```python
from build123d import *

# Parameters (mm, degrees)
F1_DEPTH = 26
F3_DEPTH = 2


with BuildPart() as f1:
    # F0 (on Top) → F1 (new body, symmetric)
    with BuildSketch(Plane.XY):
        with BuildLine():
            Line((-21.6270365771, 1), (-21.6270365771, 0))
            Line((-21.6270365771, 0), (-13.1270365771, 0))
            ThreePointArc((-13.1270365771, 0), (1.3729634229, 14.5), (15.8729634229, 0))
            Line((15.8729634229, 0), (24.3729634229, 0))
            Line((24.3729634229, 0), (24.3729634229, 1))
            Line((24.3729634229, 1), (16.8729634229, 1))
            ThreePointArc((16.8729634229, 1), (1.3729634229, 15.532224567), (-14.1270365771, 1))
            Line((-14.1270365771, 1), (-21.6270365771, 1))
        make_face()
    extrude(amount=F1_DEPTH, both=True)

    # F2 (on face) → F3 (join)
    with BuildSketch(Plane.XY.offset(26)):
        with BuildLine():
            ThreePointArc((-13.1270365771, 0), (1.3729634229, 14.5), (15.8729634229, 0))
            Line((15.8729634229, 0), (24.3729634229, 0))
            Line((24.3729634229, 0), (24.3729634229, 1))
            Line((24.3729634229, 1), (16.8729634229, 1))
            ThreePointArc((16.8729634229, 1), (1.3729634229, 15.532224567), (-14.1270365771, 1))
            Line((-14.1270365771, 1), (-21.6270365771, 1))
            Line((-21.6270365771, 1), (-21.6270365771, 0))
            Line((-21.6270365771, 0), (-13.1270365771, 0))
        make_face()
        with BuildLine():
            ThreePointArc((-1.6270365771, 0), (1.3729634229, 3), (4.3729634229, 0))
            Line((4.3729634229, 0), (15.8729634229, 0))
            ThreePointArc((15.8729634229, 0), (1.3729634229, 14.5), (-13.1270365771, 0))
            Line((-13.1270365771, 0), (-1.6270365771, 0))
        make_face()
    extrude(amount=F3_DEPTH)


solid = f1.part
```
Verification items for the finished model (mm, model axes). A direction names the side the tool comes from. Coordinates: 2 decimals unless noted, no trailing zeros. Loops run counter-clockwise (first coordinate to the right, second up) from the corner with the lowest first, then second, coordinate; pieces in that order, holes last. Notation, with made-up numbers: (58, 71) - (64, 71) arc R23 cw to (64, 92) - close; hole circle Ø5 at (87.5, 17). An arc over 180 degrees is marked (long way). Answer as a JSON object with one key per item and string values.
(1) Go/stop test with flat-tipped pins: pin 1 Ø10 at (x, z) = (-14.5, 14.5) entering from +Y; pin 2 Ø3 at (y, z) = (13.5, -1.5) entering from -X; pin 3 Ø8 at (x, z) = (21, 4.5) entering from +Y. Record where each tip stops, or that it passes through.
Response:
{"pin 1": "stops at y = 11.09", "pin 2": "stops at x = -8.49", "pin 3": "stops at y = 1"}
(2) Cross-section at D-D, the plane x = 11.5. Record the boundary of the cut face in (y, z), then the cut area to 3 significant figures.
Response:
{"outline": "(0, 26) - (10.38, 26) - (10.38, -26) - (11.78, -26) - (11.78, 28) - (0, 28) - close", "area": "96.3 mm²"}
(3) Cross-section at B-B, the plane y = 6. Record the boundary of the cut face in (x, z).
Response:
{"outline": "(-12.95, -26) - (-11.83, -26) - (-11.83, 26) - (14.57, 26) - (14.57, -26) - (15.7, -26) - (15.7, 28) - (-12.95, 28) - close"}
(4) Cross-section at C-C, the plane x = 18. Record the boundary of the cut face in (y, z).
Response:
{"outline": "(0, -26) - (1, -26) - (1, 28) - (0, 28) - close"}
(5) Mould release check, pull along X, two halves, no side actions. Record for faces 4 (the flat face through (-18, 1, 1)), 5 (the cylindrical face through (1.3, 3, 27)), 6 (the cylindrical face through (1.7, 15.53, 0.62)): pulls with the +X half, pulls with the -X half, needs draft (parallel to the pull), parting line crosses it, or undercut.
Response:
{"face 4": "needs draft", "face 5": "undercut", "face 6": "parting line crosses it"}
(6) Access from +Z, -Z, +X, -X, +Y, -Y to the whole of each face (thin tool, end or side, straight path). Record for faces 1 (the flat face through (21, 1, 1)), 2 (the flat face through (1, 6, 28)), 3 (the cylindrical face through (1.054, 14.496, 0.364)).
Response:
{"face 1": "+Z, -Z, +X, +Y", "face 2": "+Z, +X, -X, +Y, -Y", "face 3": "-Z, -Y"}
(7) Scan lines: line 1 along Z through (x, y) = (-1.5, 14); line 2 along X through (y, z) = (3.75, -6); line 3 along X through (y, z) = (4.25, 12). Record each from-to range of solid material in increasing order.
Response:
{"line 1": "z = 26 to 28", "line 2": "x = -13.7 to -12.63, 15.38 to 16.45", "line 3": "x = -13.57 to -12.49, 15.24 to 16.31"}
(8) Cross-section at A-A, the plane z = 19.5. Record the boundary of the cut face in (x, y), then the cut area to 3 significant figures.
Response:
{"outline": "(-21.63, 0) - (-13.13, 0) arc R14.5 cw to (15.87, 0) - (24.37, 0) - (24.37, 1) - (16.87, 1) arc R15.53 ccw to (-14.13, 1) - (-21.63, 1) - close", "area": "63.7 mm²"}
